```python
from build123d import *

# Parameters (mm, degrees)
SKETCH_1_W      = 29.04066115
SKETCH_1_H      = 16.7
EXTRUDE_3_DEPTH = 23.5
SKETCH_3_R      = 15
EXTRUDE_4_DEPTH = 50


with BuildPart() as part:
    # 草图1 → 凸台-拉伸3 (new body)
    with BuildSketch(Plane.XY):
        Rectangle(SKETCH_1_W, SKETCH_1_H)
        with BuildLine():
            Line((-14.520330575, -8.35), (-14.520330575, 8.35))
            ThreePointArc((-14.520330575, 8.35), (-16.75, 0), (-14.520330575, -8.35))
        make_face()
        with BuildLine():
            Line((14.520330575, -8.35), (14.520330575, 8.35))
            ThreePointArc((14.520330575, 8.35), (16.75, 0), (14.520330575, -8.35))
        make_face()
    extrude(amount=-EXTRUDE_3_DEPTH)

    # 草图3 → 凸台-拉伸4 (add)
    with BuildSketch(Plane.XY):
        with Locations(Location((0, 0, 0), (0, 0, 146.174412464))):
            Circle(SKETCH_3_R)
    extrude(amount=EXTRUDE_4_DEPTH)


solid = part.part
```
Can you work these out from the model? Positions are in its coordinate system, mm. A direction names the side the tool comes from. Give positions to 0.01 mm unless a question says otherwise; leave off trailing zeros. Loops run counter-clockwise (first coordinate to the right, second up) from the corner with the lowest first, then second, coordinate; pieces in that order, holes last. Notation, with made-up numbers: M 50.25,30 L 96.25,30 A7 ccw 96.25,38 Z; hole C 52.25,41 d8. An arc over 180 degrees is marked long. Use CSV: the item, a comma, the result in double quotes. Start each with the question number.
1. Imagine slicing it at A-A, the plane y = 0. Write out the boundary of the cut face in (x, z), plus the area to 3 significant figures.
2. Imagine slicing it at C-C, the plane z = 39.5. Write out the boundary of the cut face in (x, y), plus the area to 3 significant figures.
3. If I drill on L1, parallel to Y at x = -13.5, z = -10; L2, parallel to Y at x = 0.5, z = 2; L3, parallel to Z at x = -9.5, y = -11.5, over which ranges is the centre line in solid material (lowest first)?
4. Imagine slicing it at B-B, the plane x = 0. Write out the boundary of the cut face in (y, z), plus the area to 3 significant figures.
5. For P1, Ø8, axis at y = -2, z = 8.5, coming from the +X side; P2, Ø3.5, axis at x = -3, y = -10.5, coming from the -Z side; P3, Ø7, axis at x = -5.5, z = -12, coming from the +Y side, each with a flat end and sliding along its axis, tell me the tip position at first contact or that it passes through.
6. On a 3-axis mill with a long thin cutter (end or side, diameter ignored), from which of +Z, -Z, +X, -X, +Y, -Y can I reach the whole of each face in a straight line? I mean faces 1 (the face through (1, -12, 0)), 2 (the face through (0, 8.35, -12)), 3 (the face through (-8.31, 12.49, 24.65)). Say none if no direction works.
Response values:
1,outline,"M -16.75,-23.5 L 16.75,-23.5 L 16.75,0 L 15,0 L 15,50 L -15,50 L -15,0 L -16.75,0 Z"
1,area,"2,290 mm^2"
2,outline,"C 0,0 d30"
2,area,"707 mm^2"
3,L1,"-8.35 to 8.35"
3,L2,"-14.99 to 14.99"
3,L3,"0 to 50"
4,outline,"M -15,0 L -8.35,0 L -8.35,-23.5 L 8.35,-23.5 L 8.35,0 L 15,0 L 15,50 L -15,50 Z"
4,area,"1,890 mm^2"
5,P1,"x = 15"
5,P2,"z = 0"
5,P3,"y = 8.35"
6,face 1,"-Z, +X, -X, -Y"
6,face 2,"-Z, +X, -X, +Y"
6,face 3,"+Z"
